The model under review builds one solid part; all positions refer to its coordinate system, in mm. Face numbers are marked on the shaded views. A direction names the side the tool comes from. Round coordinates to 2 decimals unless told otherwise and drop trailing zeros. Order: outer loops, then holes, each group sorted by start corner. A loop starts at its lowest first (then second) coordinate and runs counter-clockwise, first axis right, second up. Notation, with made-up numbers: M 49.5,-35.75 L 66.5,-35.75 A11 ccw 66.5,-23.75 Z; hole C 53,57.5 d10. An arc over 180 degrees is marked long. Answer as a JSON object with one key per item and string values. Group by question number.
1. Add section D-D on x = 25. State the section outline as (y, z) points, and give its area (3 significant figures).
2. Mouldability with a two-part tool opening along X and no side actions: class the marked faces 1, 2 and 3 as released by +X, released by -X, zero draft, split by the parting line, or undercut.
3. Clearance check with flat-ended pins moving along their axes: P1, Ø6, axis at x = 25, z = -8.5, coming from the +Y side; P2, Ø3, axis at x = -10.5, y = 8.5, coming from the -Z side; P3, Ø4, axis at y = 22, z = 7, coming from the -X side; P4, Ø8, axis at x = 16.5, z = 10.5, coming from the +Y side. State where each tip first meets the part, or that it passes through.
4. Add section B-B on z = -22.5. State the section outline as (x, y) points, and give its area (3 significant figures).
5. Machinability: for the marked faces 4 and 5, which of the approach directions +Z, -Z, +X, -X, +Y, -Y give a long, thin tool a straight path to every point of the face, cutting with its end or side? Answer none if there is none.
6. To check wall thickness, follow probe 1 along X at (y, z) = (4.75, 22); probe 2 along Y at (x, z) = (7, -13); probe 3 along X at (y, z) = (17.75, -9). State the ranges of each line that lie inside material, in increasing order. Write a range as [from, to].
7. Add section C-C on y = 9.75. State the section outline as (x, z) points.
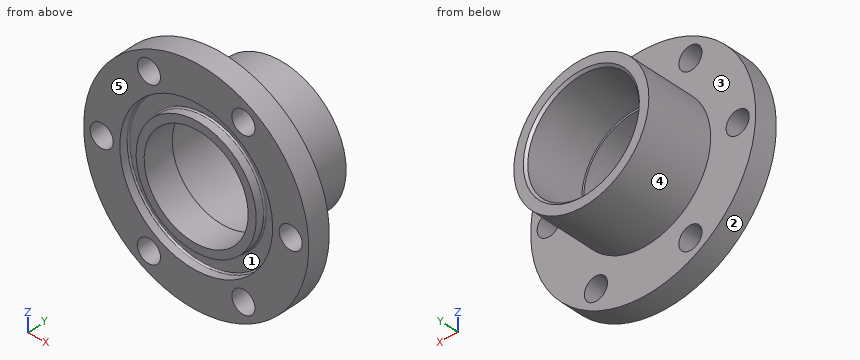
```python
from build123d import *

# Parameters (mm, degrees)
F_1_4_CLEARANCE_HOLE1_D = 6.5278
CIRPATTERN1_COUNT       = 6


with BuildPart() as part:
    # Sketch4 → Revolve1 (revolve)
    with BuildSketch(Plane.XY, mode=Mode.PRIVATE) as revolve1_sk:
        with BuildLine():
            Line((0, 25.4), (19.05, 25.4))
            Line((19.05, 25.4), (19.05, 6.35))
            Line((19.05, 6.35), (31.75, 6.35))
            Line((31.75, 6.35), (31.75, 0))
            Line((31.75, 0), (21.5773, 0))
            Line((21.5773, 0), (21.5773, 2.2606))
            ThreePointArc((21.5773, 2.2606), (21.465707684, 2.530007684), (21.1963, 2.6416))
            Line((21.1963, 2.6416), (17.3355, 2.6416))
            ThreePointArc((17.3355, 2.6416), (17.066092316, 2.530007684), (16.9545, 2.2606))
            Line((16.9545, 2.2606), (16.9545, 0))
            Line((16.9545, 0), (0, 0))
            Line((0, 0), (0, 25.4))
        make_face()
    revolve(revolve1_sk.sketch.rotate(Axis((0, 0, 0), (0, 1, 0)), 90), axis=Axis((0, 0, 0), (0, 1, 0)))

    # Sketch6 → 1 NPT Tapped Hole2 (revolve, cut)
    with BuildSketch(Plane(origin=(0, 25.4, 0), x_dir=(0, 0, 1), z_dir=(1, 0, 0))):
        Polygon((0, 0), (0, 25.4), (14.684375, 25.4), (14.684375, 16.764), (15.247532824, 16.764), (15.7299152, 0.6530848), (16.383, 0), align=None)
    revolve(axis=Axis((0, 31.75, 0), (0, -1, 0)), mode=Mode.SUBTRACT)

    # 1/4 Clearance Hole1 (through all)
    with Locations(Plane(origin=(0, 6.35, 0), x_dir=(1, 0, 0), z_dir=(0, 1, 0))):
        with Locations((26.67, 0)):
            f_1_4_clearance_hole1 = Hole(F_1_4_CLEARANCE_HOLE1_D / 2)

    # CirPattern1: 1/4 Clearance Hole1 ×6 about axis
    cirpattern1_axis = Axis((0, 0, 0), (0, 1, 0))
    for i in range(1, CIRPATTERN1_COUNT):
        add(f_1_4_clearance_hole1.rotate(cirpattern1_axis, i * 360 / CIRPATTERN1_COUNT), mode=Mode.SUBTRACT)


solid = part.part
```
Recorded:
{
 "1": {"outline": "M 0,-19.57 L 6.35,-19.57 L 6.35,-2.8 L 0,-2.8 Z; M 0,2.8 L 6.35,2.8 L 6.35,19.57 L 0,19.57 Z", "area": "213 mm²"},
 "2": {"face 1": "undercut", "face 2": "split by the parting line", "face 3": "zero draft"},
 "3": {"P1": "stops at y = 6.35", "P2": "stops at z = -16.79", "P3": "stops at x = -18.38", "P4": "stops at y = 25.4"},
 "4": {"outline": "M -22.4,0 L -16.54,0 L -16.54,6.35 L -22.4,6.35 Z; M -10.13,0 L 10.13,0 L 10.13,6.35 L -10.13,6.35 Z; M 16.54,0 L 22.4,0 L 22.4,6.35 L 16.54,6.35 Z", "area": "203 mm²"},
 "5": {"face 4": "+Y", "face 5": "+Z, -Z, +X, -X, -Y"},
 "6": {"probe 1": "x = [-22.89, -16.41], [-10.26, 10.26], [16.41, 22.89]", "probe 2": "y = [0, 8.64]", "probe 3": "x = [-16.79, -12.64], [12.64, 16.79]"},
 "7": {"outline": "C 0,0 d38.1; hole C 0,0 d30.56"}
}
